Source: CAD feature listing. Evaluate the final solid. Frame: model axes, mm. A direction names the side the tool comes from. Give positions to 0.01 mm unless a question says otherwise; leave off trailing zeros. Loops run counter-clockwise (first coordinate to the right, second up) from the corner with the lowest first, then second, coordinate; pieces in that order, holes last.
from build123d import *

# Parameters (mm, degrees)
CUT_EXTRUDE_1_REACH      = 61.305
CUT_EXTRUDE_1_END_RADIUS = 32.25
SKETCH_3_R               = 2.9
CUT_EXTRUDE_2_DEPTH      = 60.30535389
PATTERN_CIRCULAR_1_COUNT = 3
CUT_EXTRUDE_5_DEPTH      = 8.5
HOLE_WIZARD_3_8_1_D      = 10.31748
HOLE_WIZARD_3_8_1_DEPTH  = 10
HOLE_WIZARD_3_8_1_TIP    = 3.09968371
CHAMFER_1_SIZE           = 1


with BuildPart() as part:
    # 草圖1 → 旋轉1 (revolve)
    with BuildSketch(Plane.XY, mode=Mode.PRIVATE) as revolve_1_sk:
        Polygon((0, 15), (0, 0), (35.75, 0), (35.75, 31), (27.75, 31), (27.75, 15), align=None)
    revolve(revolve_1_sk.sketch.rotate(Axis((0, 38.135683761, 0), (0, -1, 0)), 180), axis=Axis((0, 38.135683761, 0), (0, -1, 0)))

    # 除料-伸長1: up to this cylinder (the profile starts inside it)
    cut_extrude_1_end = Plane(origin=(0, 23, 0), z_dir=(0, 1, 0)) * Cylinder(CUT_EXTRUDE_1_END_RADIUS, 188.11, mode=Mode.PRIVATE)
    # 草圖2 → 除料-伸長1 (cut, up to the surface)
    with BuildSketch(Plane(origin=(0, 0, 0), x_dir=(0, 0, -1), z_dir=(1, 0, 0)), mode=Mode.PRIVATE) as cut_extrude_1_sk1:
        Polygon((0, 27.618802154), (-4, 25.309401077), (-4, 20.690598923), (0, 18.381197846), (4, 20.690598923), (4, 25.309401077), align=None)
    cut_extrude_1_tool1 = extrude(cut_extrude_1_sk1.sketch, amount=CUT_EXTRUDE_1_REACH, mode=Mode.PRIVATE) & cut_extrude_1_end
    cut_extrude_1 = cut_extrude_1_tool1.solids().sort_by_distance((0, 23, 0))[0]
    add(cut_extrude_1, mode=Mode.SUBTRACT)

    # 草圖3 → 除料-伸長2 (cut, through all)
    with BuildSketch(Plane(origin=(0, 0, 0), x_dir=(0, 0, -1), z_dir=(1, 0, 0))):
        with Locations(Location((0, 23, 0), (0, 0, 180))):
            Circle(SKETCH_3_R)
    cut_extrude_2 = extrude(amount=CUT_EXTRUDE_2_DEPTH, mode=Mode.SUBTRACT)

    # 環狀複製排列1: 除料-伸長1, 除料-伸長2 ×3 about axis
    pattern_circular_1_axis = Axis((0, 0, 0), (0, 1, 0))
    add([cut_extrude_1.rotate(pattern_circular_1_axis, i * 360 / PATTERN_CIRCULAR_1_COUNT) for i in range(1, PATTERN_CIRCULAR_1_COUNT)], mode=Mode.SUBTRACT)
    add([cut_extrude_2.rotate(pattern_circular_1_axis, i * 360 / PATTERN_CIRCULAR_1_COUNT) for i in range(1, PATTERN_CIRCULAR_1_COUNT)], mode=Mode.SUBTRACT)

    # 草圖6 → 除料-伸長5 (cut)
    with BuildSketch(Plane(origin=(0, 15, 0), x_dir=(1, 0, 0), z_dir=(0, 1, 0))):
        Polygon((8.082903769, 0), (4.041451884, 7), (-4.041451884, 7), (-8.082903769, 0), (-4.041451884, -7), (4.041451884, -7), align=None)
    extrude(amount=-CUT_EXTRUDE_5_DEPTH, mode=Mode.SUBTRACT)

    # 3/8 餘隙孔1
    with Locations(Plane(origin=(0, 0, 0), x_dir=(-1, 0, 0), z_dir=(0, -1, 0))):
        with Locations((0, 0)):
            Hole(HOLE_WIZARD_3_8_1_D / 2, depth=HOLE_WIZARD_3_8_1_DEPTH)
            with Locations((0, 0, -(HOLE_WIZARD_3_8_1_DEPTH + HOLE_WIZARD_3_8_1_TIP / 2))):  # 118° drill point
                Cone(0, HOLE_WIZARD_3_8_1_D / 2, HOLE_WIZARD_3_8_1_TIP, mode=Mode.SUBTRACT)

    # 導角1
    chamfer_1_edges = [part.edges().sort_by_distance(p)[0] for p in [
        (27.75, 31, 0),
    ]]
    chamfer(chamfer_1_edges, length=CHAMFER_1_SIZE)


solid = part.part
1) Cut plane C-C (y = 24). Return loops of the section in (x, z), and give its area (3 significant figures).
Checks:
outline: (-20.18, -29.51) - (-18.42, -26.47) arc R32.25 cw to (-19.46, -25.71) - (-17.19, -21.78) arc R27.75 cw to (-17.19, 21.78) - (-19.46, 25.71) arc R32.25 cw to (-18.42, 26.47) - (-20.18, 29.51) arc R35.75 ccw to start; (-15.47, -32.23) arc R35.75 ccw to (35.65, -2.72) - (32.13, -2.72) arc R32.25 cw to (32, -4) - (27.46, -4) arc R27.75 cw to (-10.27, -25.78) - (-12.54, -29.71) arc R32.25 cw to (-13.71, -29.19) - close; (-15.47, 32.23) - (-13.71, 29.19) arc R32.25 cw to (-12.54, 29.71) - (-10.27, 25.78) arc R27.75 cw to (27.46, 4) - (32, 4) arc R32.25 cw to (32.13, 2.72) - (35.65, 2.72) arc R35.75 ccw to start
area: 1,430 mm2
2) Contact query for flat-ended pins moving along their axis: P1, Ø3, axis at x = -20.5, y = 15.5, coming from the +Z side; P2, Ø8, axis at y = 9.5, z = 18.5, coming from the +X side; P3, Ø8, axis at x = 12.5, y = 14, coming from the -Z side. Output: stop coordinate, or through.
Checks:
P1: stops at z = 30.28
P2: stops at x = 32.68
P3: stops at z = -34.72
3) Ray query, probe 1 along Z at (x, y) = (0, 24); probe 2 along Y at (x, z) = (33.45, 0); probe 3 along X at (y, z) = (24, -7). Return the intervals inside material, ascending.
Checks:
probe 1: z = -35.75 to -27.75, 27.75 to 35.75
probe 2: y = 0 to 20.1, 25.9 to 31
probe 3: x = -35.06 to -26.85, 26.85 to 35.06
4) Cut plane D-D (y = 4.5). Return loops of the section in (x, z).
Checks:
outline: circle Ø71.5 at (0, 0); hole circle Ø10.32 at (0, 0)
5) Cut plane A-A (x = 0). Return loops of the section in (y, z), and give its area (3 significant figures).
Checks:
outline: (0, -35.75) - (31, -35.75) - (31, -28.75) - (30, -27.75) - (15, -27.75) - (15, -7) - (6.5, -7) - (6.5, -5.16) - (0, -5.16) - close; (0, 5.16) - (6.5, 5.16) - (6.5, 7) - (15, 7) - (15, 27.75) - (30, 27.75) - (31, 28.75) - (31, 35.75) - (0, 35.75) - close
area: 1,140 mm2
6) Pull-direction query (Z, two-part tool) for faces 1 (the flat face through (-1, 0, 7)), 2 (the flat face through (29.82, 26.48, 1.97)), 3 (the cylindrical face through (26.35, 15.72, -24.16)), 4 (the flat face through (-13.2, 19.52, 26.81)); classes: released by +Z, released by -Z, zero draft, split by the parting line, or undercut.
Checks:
face 1: zero draft
face 2: undercut
face 3: split by the parting line
face 4: undercut
7) Cut plane B-B (y = 12). Return loops of the section in (x, z).
Checks:
outline: circle Ø71.5 at (0, 0); hole (-8.08, 0) - (-4.04, -7) - (4.04, -7) - (8.08, 0) - (4.04, 7) - (-4.04, 7) - close
8) Reachability of faces 5 (the cylindrical face through (-15.3, 19.99, -28.39)), 6 (the flat face through (0, 11, -7)), 7 (the cylindrical face through (-1.118, 3.296, 5.036)) from +Z, -Z, +X, -X, +Y, -Y: full face, straight path, thin tool, end or side. Return the list, or none.
Checks:
face 5: none
face 6: +Y
face 7: +Y, -Y
